Model file for the job. Use its own axes, mm. A direction names the side the tool comes from. Coordinates: 2 decimals unless noted, no trailing zeros. Write each loop counter-clockwise with the first axis right and the second up, starting at its lowest first coordinate (ties: lowest second). Pieces come first, ordered by that corner, then holes. Notation, with made-up numbers: M 88,81.25 L 103,81.25 A28 cw 103,117.25 Z; hole C 13,9 d2. An arc over 180 degrees is marked long. One line per question, with ' | ' between items. Start each with the question number.
(1) Flat gauge pins, fed straight in: pin 1 Ø2 at (y, z) = (32.5, -7.5) entering from -X; pin 2 Ø4 at (x, z) = (7.5, -22.5) entering from +Y; pin 3 Ø1 at (y, z) = (32, -4) entering from -X; pin 4 Ø4 at (y, z) = (32.5, -22.5) entering from -X. Where does each tip first touch, or does it go through?
(2) Tool access for faces 4 (the face through (21, 4, -6)), 5 (the face through (0, 5, -15)), 6 (the face through (32.958, 19.697, -9.895)), 7 (the face through (37.97, 18.68, -23.79)), 8 (the face through (30, 25, -15)): list every direction of +Z, -Z, +X, -X, +Y, -Y with a clear straight run to the whole face (end or side of a thin tool).
(3) Cut at B-B (y = 17.5). Write the cut outline in (x, z), plus the area to 3 significant figures.
(4) Two-plate mould, pull along X, no slides. Class faces 1 (the face through (36, 16, -21)), 2 (the face through (38, 34, -6.6)), 3 (the face through (7.58, 2.03, -24.25)): +X half, -X half, draft (parallel to the pull), parting line (faces both ways), or undercut.
(5) Cut at D-D (z = -22.5). Count the separate pieces of the cut face and the enclosed holes in it, plus the area to 3 significant figures.
(6) Wall check: probe 1 along Y at (x, z) = (39, -22.5); probe 2 along X at (y, z) = (8.05, -7.5); probe 3 along X at (y, z) = (0.95, -22.5). Give the ranges that are in metal, low to high.
(7) Cut at A-A (x = 37.5). Write the cut outline in (y, z), plus the area to 3 significant figures.
(8) Cut at C-C (x = 7.5). Write the cut outline in (y, z).
from build123d import *

# Parameters (mm, degrees)
ESBO_O1_W                = 40
ESBO_O1_H                = 30
RESSALTO_EXTRUS_O1_DEPTH = 10
ESBO_O2_W                = 10
ESBO_O2_H                = 30
RESSALTO_EXTRUS_O2_DEPTH = 30
ESBO_O4_R                = 3.25
CORTE_EXTRUS_O1_DEPTH    = 6
ESBO_O5_R                = 1.75
CORTE_EXTRUS_O2_DEPTH    = 10
ESBO_O6_R                = 3.25
CORTE_EXTRUS_O3_DEPTH    = 6
ESBO_O7_R                = 1.75
CORTE_EXTRUS_O4_DEPTH    = 10


with BuildPart() as part:
    # Esboço1 → Ressalto-extrusão1 (new body)
    with BuildSketch(Plane(origin=(0, 0, 0), x_dir=(1, 0, 0), z_dir=(0, 1, 0))):
        with Locations((20, 15)):
            Rectangle(ESBO_O1_W, ESBO_O1_H)
    extrude(amount=RESSALTO_EXTRUS_O1_DEPTH)

    # Esboço2 → Ressalto-extrusão2 (add)
    with BuildSketch(Plane(origin=(0, 10, 0), x_dir=(1, 0, 0), z_dir=(0, 1, 0))):
        with Locations((35, 15)):
            Rectangle(ESBO_O2_W, ESBO_O2_H)
    extrude(amount=RESSALTO_EXTRUS_O2_DEPTH)

    # Esboço4 → Corte-extrusão1 (cut)
    with BuildSketch(Plane(origin=(0, 10, 0), x_dir=(1, 0, 0), z_dir=(0, 1, 0))):
        with Locations(Location((7.5, 22.5, 0), (0, 0, 270))):
            Circle(ESBO_O4_R)
        with Locations(Location((22.5, 22.5, 0), (0, 0, 270))):
            Circle(ESBO_O4_R)
        with Locations(Location((22.5, 7.5, 0), (0, 0, 270))):
            Circle(ESBO_O4_R)
        with Locations(Location((7.5, 7.5, 0), (0, 0, 270))):
            Circle(ESBO_O4_R)
    extrude(amount=-CORTE_EXTRUS_O1_DEPTH, mode=Mode.SUBTRACT)

    # Esboço5 → Corte-extrusão2 (cut)
    with BuildSketch(Plane(origin=(0, 10, 0), x_dir=(1, 0, 0), z_dir=(0, 1, 0))):
        with Locations(Location((7.5, 22.5, 0), (0, 0, 270))):
            Circle(ESBO_O5_R)
        with Locations(Location((22.5, 22.5, 0), (0, 0, 270))):
            Circle(ESBO_O5_R)
        with Locations(Location((22.5, 7.5, 0), (0, 0, 270))):
            Circle(ESBO_O5_R)
        with Locations(Location((7.5, 7.5, 0), (0, 0, 270))):
            Circle(ESBO_O5_R)
    extrude(amount=-CORTE_EXTRUS_O2_DEPTH, mode=Mode.SUBTRACT)

    # Esboço6 → Corte-extrusão3 (cut)
    with BuildSketch(Plane.ZY.offset(-30)):
        with Locations((-7.5, 32.5)):
            Circle(ESBO_O6_R)
        with Locations((-22.5, 32.5)):
            Circle(ESBO_O6_R)
        with Locations((-22.5, 17.5)):
            Circle(ESBO_O6_R)
        with Locations((-7.5, 17.5)):
            Circle(ESBO_O6_R)
    extrude(amount=-CORTE_EXTRUS_O3_DEPTH, mode=Mode.SUBTRACT)

    # Esboço7 → Corte-extrusão4 (cut)
    with BuildSketch(Plane.ZY.offset(-30)):
        with Locations((-22.5, 32.5)):
            Circle(ESBO_O7_R)
        with Locations((-7.5, 32.5)):
            Circle(ESBO_O7_R)
        with Locations((-7.5, 17.5)):
            Circle(ESBO_O7_R)
        with Locations((-22.5, 17.5)):
            Circle(ESBO_O7_R)
    extrude(amount=-CORTE_EXTRUS_O4_DEPTH, mode=Mode.SUBTRACT)


solid = part.part
Filled in:
1) pin 1: through | pin 2: y = 4 | pin 3: x = 30 | pin 4: x = 36
2) face 4: +Y | face 5: +Z, -Z, -X, +Y, -Y | face 6: -X | face 7: +X, -X | face 8: +Z, -Z, -X, +Y
3) outline: M 30,-30 L 40,-30 L 40,-24.25 L 36,-24.25 L 36,-25.75 L 30,-25.75 Z; M 30,-19.25 L 36,-19.25 L 36,-20.75 L 40,-20.75 L 40,-9.25 L 36,-9.25 L 36,-10.75 L 30,-10.75 Z; M 30,-4.25 L 36,-4.25 L 36,-5.75 L 40,-5.75 L 40,0 L 30,0 Z | area: 194 mm²
4) face 1: -X half | face 2: draft | face 3: undercut
5) separate pieces: 5 | enclosed holes: 0 | area: 488 mm²
6) probe 1: 0 to 15.75, 19.25 to 30.75, 34.25 to 40 | probe 2: 0 to 4.25, 10.75 to 19.25, 25.75 to 40 | probe 3: 0 to 5.75, 9.25 to 20.75, 24.25 to 40
7) outline: M 0,-30 L 40,-30 L 40,0 L 0,0 Z; hole C 17.5,-22.5 d3.5; hole C 17.5,-7.5 d3.5; hole C 32.5,-22.5 d3.5; hole C 32.5,-7.5 d3.5 | area: 1,160 mm²
8) outline: M 0,-30 L 10,-30 L 10,-25.75 L 4,-25.75 L 4,-24.25 L 0,-24.25 Z; M 0,-20.75 L 4,-20.75 L 4,-19.25 L 10,-19.25 L 10,-10.75 L 4,-10.75 L 4,-9.25 L 0,-9.25 Z; M 0,-5.75 L 4,-5.75 L 4,-4.25 L 10,-4.25 L 10,0 L 0,0 Z
